The model under review builds one solid part; all positions refer to its coordinate system, in mm. A direction names the side the tool comes from. Round coordinates to 2 decimals unless told otherwise and drop trailing zeros. Order: outer loops, then holes, each group sorted by start corner. A loop starts at its lowest first (then second) coordinate and runs counter-clockwise, first axis right, second up. Notation, with made-up numbers: (41.25, 8) -> (78.25, 8) arc R11 cw to (78.25, 28) -> close; hole circle Ø9 at (-7.75, 2). An arc over 180 degrees is marked (long way). Put each result on its own line as item: value. Start each with the question number.
Autodesk Inventor part; units mm, degrees
ref_plane "YZ Plane" through (0, 0, 0) normal (1, 0, 0) x (0, 1, 0)
ref_plane "XZ Plane" through (0, 0, 0) normal (0, 1, 0) x (-1, 0, 0)
ref_plane "XY Plane" through (0, 0, 0) normal (0, 0, 1) x (1, 0, 0)
sketch "Sketch1" plane through (0, 0, 0) normal (0, 0, 1) x (1, 0, 0)
  line L0 (-25.4, 25.4) -> (25.4, 25.4)
  line L1 (25.4, 25.4) -> (25.4, -25.4)
  line L2 (25.4, -25.4) -> (-25.4, -25.4)
  line L3 (-25.4, -25.4) -> (-25.4, 25.4)
  line L4 (19.05, 19.05) -> (-19.05, 19.05)
  line L5 (-19.05, 19.05) -> (-19.05, -19.05)
  line L6 (-19.05, -19.05) -> (19.05, -19.05)
  line L7 (19.05, -19.05) -> (19.05, 19.05)
  circle A0 centre (0, 0) radius 9.525
  point P0 (0, 25.4)
  point P1 (-25.4, 0)
  dimension "d0" = 50.8
  dimension "d1" = 50.8
  dimension "d2" = 6.35
  dimension "d20" = 19.05
extrude "Extrusion1" add sketch "Sketch1" along normal mid plane 711.2 contours L0 L1 L2 L3
extrude "Extrusion4" add sketch "Sketch1" along normal mid plane 50.8 contours L7 L6 L5 L4
sketch "Sketch2" plane through (25.4, -25.4, 355.6) normal (1, 0, 0) x (0, 0, -1)
  line L0 (711.2, 0) -> (711.2, 50.8)
  circle A0 centre (673.1, 25.4) radius 14.2875
  line L1 (0, 50.8) -> (0, 0)
  circle A1 centre (76.2, 25.4) radius 14.2875
  point P0 (355.6, 25.4)
  point P1 (711.2, 25.4)
  point P2 (0, 25.4)
  dimension "d5" = 28.575
  dimension "d6" = 38.1
  dimension "d18" = 76.2
extrude "Extrusion2" cut sketch "Sketch2" against normal up to surface (50.8 mm away)
sketch "Sketch3" plane through (25.4, -25.4, 355.6) normal (1, 0, 0) x (0, 0, -1)
  line L0 (0, 0) -> (711.2, 0)
  line L1 (0, 50.8) -> (711.2, 50.8)
  arc A0 (-101.6, 139.7) -> (-101.6, 88.9) centre (-101.6, 114.3) ccw
  circle A1 centre (-101.6, 114.3) radius 14.2875
  line L2 (-101.6, 88.9) -> (-25.4, 88.9)
  line L3 (-101.6, 139.7) -> (50.8, 139.7)
  line L4 (0, 50.8) -> (0, 63.5)
  line L5 (76.2, 114.3) -> (76.2, 50.8)
  arc A2 (76.2, 114.3) -> (50.8, 139.7) centre (50.8, 114.3) ccw
  arc A3 (0, 63.5) -> (-25.4, 88.9) centre (-25.4, 63.5) ccw
  point P0 (355.6, 25.4)
  point P1 (0, 88.9)
  point P2 (76.2, 139.7)
  dimension "d9" = 28.575
  dimension "d10" = 25.4
  dimension "d11" = 101.6
  dimension "d12" = 76.2
  dimension "d13" = 38.1
  dimension "d14" = 25.4
extrude "Extrusion3" add sketch "Sketch3" against normal up to surface (50.8 mm away)
properties part number "Arm"
Q1. Take a section at A-A on y = 0. State how many separate pieces and enclosed holes the cut face has, and give its area (3 significant figures).
Q2. Clearance check with flat-ended pins moving along their axes: pin 1 Ø23 at (y, z) = (0, 279.4) entering from -X; pin 2 Ø2 at (x, y) = (-16, 39) entering from +Z; pin 3 Ø15 at (x, y) = (4.5, 67) entering from -Z; pin 4 Ø1.5 at (x, y) = (-18, 56) entering from +Z. State where each tip first meets the part, or that it passes through.
Q3. Take a section at B-B on z = -317.5. Give the boundary of the cut face in (x, y).
Q4. For faces 1 (the face through (19.05, 0, 188)), 2 (the face through (-5, 9, -25.4)), 3 (the face through (0, 114.3, 382)), list the 3-axis set-ups (+Z, -Z, +X, -X, +Y, -Y) from which the entire face can be reached by the end or side of a thin tool; tool diameter is ignored.
Q5. Wall thickness on probe 1 along Y at (x, z) = (9.5, 457.2); probe 2 along X at (y, z) = (-15.5, 239): over which ranges is each line inside the solid? List them lowest first. Write a range as [from, to].
Q6. Draft analysis for pull direction Y (two halves, no side actions). For faces 4 (the face through (0.36, 106.66, 286.64)), 5 (the face through (22.269, 0.628, -303.226)), 6 (the face through (0, 63.5, 420)), state which applies: +Y half, -Y half, draft (parallel to the pull), parting line (faces both ways), or undercut.
Q7. Take a section at D-D on z = -217. Give the boundary of the cut face in (x, y).
Calculated:
1. separate pieces: 6
1. enclosed holes: 0
1. area: 9,270 mm²
2. pin 1: passes through
2. pin 2: stops at z = 355.67
2. pin 3: stops at z = 279.4
2. pin 4: stops at z = 363.76
3. outline: (-25.4, -25.4) -> (25.4, -25.4) -> (25.4, -14.29) -> (19.05, -14.29) -> (19.05, -19.05) -> (-19.05, -19.05) -> (-19.05, -14.29) -> (-25.4, -14.29) -> close; (-25.4, 14.29) -> (-19.05, 14.29) -> (-19.05, 19.05) -> (19.05, 19.05) -> (19.05, 14.29) -> (25.4, 14.29) -> (25.4, 25.4) -> (-25.4, 25.4) -> close
4. face 1: +Z
4. face 2: -Z
4. face 3: +Z, -Z, +X, -X, +Y
5. probe 1: y = [63.5, 74.61], [103.19, 114.3]
5. probe 2: x = [-25.4, -19.05], [19.05, 25.4]
6. face 4: +Y half
6. face 5: undercut
6. face 6: -Y half
7. outline: (-25.4, -25.4) -> (25.4, -25.4) -> (25.4, 25.4) -> (-25.4, 25.4) -> close; hole (-19.05, -19.05) -> (19.05, -19.05) -> (19.05, 19.05) -> (-19.05, 19.05) -> close
